Autodesk Inventor part; units mm, degrees
ref_plane "Work Plane1" through (0, 0, 10.287) normal (0, 0, -1) x (-1, 0, 0)
ref_plane "YZ Plane" through (0, 0, 0) normal (1, 0, 0) x (0, 1, 0)
ref_plane "XZ Plane" through (0, 0, 0) normal (0, 1, 0) x (-1, 0, 0)
sketch "Sketch1" plane through (0, 0, 0) normal (0, 0, 1) x (1, 0, 0)
  line L0 (0, 0) -> (38.1, 0)
  line L1 (38.1, 0) -> (38.1, 31.4433)
  line L2 (0, 66.04) -> (0, 0)
  line L3 (0, 66.04) -> (13.5942, 73.8886)
  line L4 (0, 66.04) -> (12.7, 44.043)
  line L5 (12.7, 44.043) -> (26.2942, 51.8916)
  line L6 (26.2942, 51.8916) -> (13.5942, 73.8886)
  line L7 (26.2942, 51.8916) -> (38.1, 31.4433)
  dimension "d0" = 15.6972
  dimension "d1" = 25.4
  dimension "d2" = 38.1
  dimension "d3" = 66.04
  dimension "d4" = 120
extrude "Extrusion1" add sketch "Sketch1" along normal blind 20.574 contours L2 L4 L5 L7 L1 L0
sketch "Sketch2" plane through (0, 0, 20.574) normal (0, 0, 1) x (1, 0, 0)
  line L0 (0, 66.04) -> (0, 0)
  line L1 (0, 0) -> (38.1, 0)
  line L2 (38.1, 0) -> (38.1, 31.4433)
  line L3 (38.1, 31.4433) -> (26.2942, 51.8916)
  line L4 (26.2942, 51.8916) -> (12.7, 44.043)
  line L5 (12.7, 44.043) -> (0, 66.04)
  line L6 (26.2942, 51.8916) -> (13.5942, 73.8886)
  line L7 (13.5942, 73.8886) -> (0, 66.04)
  line L8 (38.1, 31.4433) -> (26.2942, 51.8916)
extrude "Extrusion2" add sketch "Sketch2" along normal blind 2.54
ref_plane "Work Plane1" through (0, 0, 10.287) normal (0, 0, -1) x (-1, 0, 0)
mirror "Mirror1" about plane through (0, 0, 10.287) normal (0, 0, -1) of "Extrusion2"
sketch "Sketch3" plane through (0, 0, 23.114) normal (0, -1, 0) x (1, 0, 0)
  line L0 (38.1, -25.654) -> (38.1, 0)
  line L1 (38.1, -6.477) -> (33.02, -6.477)
  line L2 (33.02, -6.477) -> (33.02, -19.177)
  line L3 (33.02, -19.177) -> (38.1, -19.177)
  line L4 (38.1, -19.177) -> (38.1, -6.477)
  point P0 (0, -23.114)
  point P1 (38.1, -12.827)
  dimension "d9" = 12.7
  dimension "d10" = 5.08
  dimension "d11" = 6.35
extrude "Extrusion3" cut sketch "Sketch3" against normal blind 111.125
sketch "Sketch4" plane through (33.02, 0, 16.637) normal (1, 0, 0) x (0, 0, -1)
  circle A0 centre (6.35, 15.042) radius 1.778
  point P0 (16.637, 0)
extrude "Extrusion4" cut sketch "Sketch4" against normal blind 15.24
sketch "Sketch5" plane through (13.5942, 73.8886, 23.114) normal (0.8660254, 0.5, 0) x (0, 0, -1)
  line L0 (23.114, -25.4) -> (2.54, -25.4)
  line L1 (23.114, -25.4) -> (2.54, -25.4)
  line L2 (2.54, -25.4) -> (2.54, -37.7698)
  line L3 (2.54, -37.7698) -> (23.114, -37.7698)
  line L4 (23.114, -37.7698) -> (23.114, -25.4)
  point P0 (23.114, -57.1923)
  dimension "d16" = 12.3698
extrude "Extrusion5" cut sketch "Sketch5" against normal blind 5.08
chamfer "Chamfer1" distance 1.016 angle 45 1 edges at (21.893, 49.3506, 10.287)
sketch "Sketch6" plane through (9.1948, 71.3486, 23.114) normal (0.8660254, 0.5, 0) x (0, 0, -1)
  line L0 (22.86, -25.4) -> (2.54, -25.4)
  line L1 (23.114, -37.7698) -> (2.54, -37.7698)
  line L2 (2.54, -25.4) -> (2.54, 0)
  line L3 (2.54, -37.7698) -> (2.54, 0)
  line L4 (2.54, -25.4) -> (2.54, -37.7698)
  circle A0 centre (12.827, -31.5849) radius 1.778
  point P0 (23.114, -57.1923)
  point P1 (2.54, -31.5849)
  point P2 (12.827, -37.7698)
  dimension "d22" = 3.556
extrude "Extrusion6" cut sketch "Sketch6" against normal blind 7.62
ref_plane "Work Plane2" through (0, 0, 10.287) normal (0, 0, 1) x (1, 0, 0)
sketch "Sketch7" plane through (0, 0, 10.287) normal (0, 0, 1) x (1, 0, 0)
  line L0 (12.7, 44.043) -> (-2.54, 70.4394)
  line L1 (21.0809, 48.8817) -> (12.7, 44.043)
  line L2 (16.51, 46.2427) -> (11.43, 46.2427)
  line L3 (11.43, 46.2427) -> (11.43, 0)
  line L4 (11.43, 0) -> (16.51, 0)
  line L5 (16.51, 0) -> (16.51, 46.2427)
  line L6 (0, 0) -> (38.1, 0)
  dimension "d25" = 5.08
extrude "Extrusion7" cut sketch "Sketch7" along normal mid plane 10.16 contours L1 L5 L4 L3 L0
ref_plane "Work Plane3" through (0, 6.35, 23.114) normal (0, -1, 0) x (1, 0, 0)
sketch "Sketch8" plane through (0, 6.35, 23.114) normal (0, -1, 0) x (1, 0, 0)
  line L0 (0, -25.654) -> (38.1, -25.654)
  line L1 (0, -25.654) -> (0, 0)
  line L2 (14.7303, -25.654) -> (17.0826, -23.0077)
  line L3 (17.0826, -23.0077) -> (0, -7.8232)
  line L4 (4.8537, -36.7652) -> (14.7303, -25.654)
  line L5 (0, -32.4508) -> (-19.3376, -15.2619)
  point P0 (0, -23.114)
  dimension "d37" = 17.8308
extrude "Extrusion8" cut sketch "Sketch8" against normal blind 12.7
sketch "Sketch9" plane through (0, 6.35, 15.2908) normal (-0.6643638, 0, -0.7474093) x (-0.7474093, 0, 0.6643638)
  line L0 (-8.4923, 39.8927) -> (-8.4923, -6.35)
  line L1 (-19.039, 39.8927) -> (-19.039, -6.35)
  line L2 (-22.8557, 0) -> (0, 0)
  line L3 (0, 12.7) -> (-22.8557, 12.7)
  point P0 (-10.1587, -6.35)
  point P1 (-8.4923, 12.7)
  point P2 (-19.039, 12.7)
  point P3 (-19.039, 0)
  point P4 (-8.4923, 0)
extrude "Extrusion9" cut sketch "Sketch9" against normal up to next
sketch "Sketch11" plane through (0, 0, 23.114) normal (-1, 0, 0) x (0, 0, 1)
  circle A0 centre (-12.827, 35.56) radius 1.778
  point P0 (-23.114, 0)
extrude "Extrusion11" cut sketch "Sketch11" against normal blind 15.24
sketch "Sketch13" plane through (0, 0, 23.114) normal (0, -1, 0) x (1, 0, 0)
  circle A0 centre (22.86, -6.35) radius 1.778
  point P0 (0, -23.114)
extrude "Extrusion13" cut sketch "Sketch13" against normal blind 15.24
sketch "Sketch14" plane through (38.1, 0, -2.54) normal (0, 0, -1) x (-1, 0, 0)
  circle A0 centre (12.7, 25.4) radius 1.778
  point P0 (38.1, 0)
extrude "Extrusion14" cut sketch "Sketch14" against normal blind 15.24
sketch "Sketch15" plane through (0, 0, 5.207) normal (0, 0, 1) x (1, 0, 0)
  line L0 (16.51, 6.35) -> (16.51, 0)
  line L1 (11.43, 0) -> (16.51, 0)
  line L2 (16.51, 0) -> (16.51, 7.62)
  line L3 (16.51, 7.62) -> (11.43, 7.62)
  line L4 (11.43, 7.62) -> (11.43, 0)
  point P0 (0, 0)
  dimension "d50" = 7.62
extrude "Extrusion15" cut sketch "Sketch15" against normal blind 12.7
properties part number "PALM 4"
CAD build for the part. Positions are in the model's coordinates, mm. A direction names the side the tool comes from. Give positions to 0.01 mm unless a question says otherwise; leave off trailing zeros. Order: outer loops, then holes, each group sorted by start corner. A loop starts at its lowest first (then second) coordinate and runs counter-clockwise, first axis right, second up. Notation, with made-up numbers: (40, 39.5) - (55, 39.5) arc R15 cw to (55, 67.5) - close; hole circle Ø9 at (-10, -9.5). An arc over 180 degrees is marked (long way). Answer in a Markdown table with one row per item.
1. Saw through at D-D, the plane x = 34. Give the cut face in (y, z).
Data:
| item | result |
|---|---|
| outline | (0, -2.54) - (38.54, -2.54) - (38.54, 3.94) - (0, 3.94) - close; (0, 16.64) - (38.54, 16.64) - (38.54, 23.11) - (0, 23.11) - close |
2. Saw through at A-A, the plane z = 1.75. Give the cut face in (x, y).
Data:
| item | result |
|---|---|
| outline | (0, 0) - (11.43, 0) - (11.43, 6.35) - (0, 6.35) - close; (0, 19.05) - (15.23, 19.05) - (15.23, 7.62) - (16.51, 7.62) - (16.51, 0) - (38.1, 0) - (38.1, 31.44) - (32.48, 41.18) - (28.08, 38.64) - (22.4, 48.47) - (21.01, 48.84) - (12.7, 44.04) - (0, 66.04) - close; hole circle Ø3.56 at (25.4, 25.4) |
3. Flat gauge pins, fed straight in: pin 1 (8.5 mm diameter, centred on x = 4.5, z = 5.5, fed in from -Y); pin 2 (3 mm diameter, centred on y = 15.042, z = 10.287, fed in from -X); pin 3 (6 mm diameter, centred on x = 17, z = 1.5, fed in from +Y); pin 4 (0.5 mm diameter, centred on x = 16, z = -2, fed in from -Y). Where does each tip first touch, or does it go through?
Data:
| item | result |
|---|---|
| pin 1 | stops at y = 0 |
| pin 2 | stops at x = 3.94 |
| pin 3 | stops at y = 72.49 |
| pin 4 | stops at y = 7.62 |
4. Saw through at C-C, the plane z = 11.25. Count the separate pieces of the cut face and the enclosed holes in it, plus the area to 3 significant figures.
Data:
| item | result |
|---|---|
| separate pieces | 3 |
| enclosed holes | 1 |
| area | 1,150 mm² |
5. Saw through at B-B, the plane y = 25.4. Give the cut face in (x, z).
Data:
| item | result |
|---|---|
| outline | (0, -2.54) - (23.62, -2.54) - (23.62, 12.7) - (27.18, 12.7) - (27.18, -2.54) - (38.1, -2.54) - (38.1, 3.94) - (33.02, 3.94) - (33.02, 16.64) - (38.1, 16.64) - (38.1, 23.11) - (0, 23.11) - close; hole (11.43, 5.21) - (16.51, 5.21) - (16.51, 15.37) - (11.43, 15.37) - close |
6. Tool access for faces 4 (the flat face through (15.89, 12.611, -1.235)), 5 (the flat face through (11.43, 3, 6)), 6 (the flat face through (17.78, 15, 10)): list every direction of +Z, -Z, +X, -X, +Y, -Y with a clear straight run to the whole face (end or side of a thin tool).
Data:
| item | result |
|---|---|
| face 4 | -X |
| face 5 | -Z, -Y |
| face 6 | +X |
7. Probe probe 1 along Z at (x, y) = (15, 46); probe 2 along Z at (x, y) = (36.5, 24); probe 3 along Y at (x, z) = (7, 11.25). List the from-to ranges inside material, lowest first. Write a range as [from, to].
Data:
| item | result |
|---|---|
| probe 1 | z = [-2.54, 0], [20.57, 23.11] |
| probe 2 | z = [-2.54, 3.94], [16.64, 23.11] |
| probe 3 | y = [0, 34.07], [37.05, 53.92] |
8. Pull direction Z, two halves, no side cores. Call faces 1 (the flat face through (19, 37, -2.54)), 2 (the flat face through (6.7, 69.91, -1.25)), 3 (the flat face through (16, 57, 20.574)): pulls with the +Z half, pulls with the -Z half, needs draft (parallel to the pull), parting line crosses it, or undercut.
Data:
| item | result |
|---|---|
| face 1 | pulls with the -Z half |
| face 2 | needs draft |
| face 3 | undercut |
